Input: part model. Units: mm. Frame: model coordinates. Coordinates: 2 decimals unless noted, no trailing zeros. Order: outer loops, then holes, each group sorted by start corner. A loop starts at its lowest first (then second) coordinate and runs counter-clockwise, first axis right, second up. Notation, with made-up numbers: (79, -13) -> (137, -13) arc R18 cw to (137, 18) -> close; hole circle Ø4 at (64.5, 86). An arc over 180 degrees is marked (long way). Answer as CSV lines item,"result".
Solid Edge part; units mm, degrees
sketch "Sketch1" plane through (0, 0, 0) normal (0, -1, 0) x (1, 0, 0)
  line L0 (-92.8835, -94.8099) -> (-82.8835, -94.8099)
  line L1 (-82.8835, -94.8099) -> (-82.8835, 45.1901)
  line L2 (-82.8835, 45.1901) -> (-92.8835, 45.1901)
  line L3 (-92.8835, 45.1901) -> (-92.8835, -94.8099)
  dimension "D1" = 82.8835
  dimension "D2" = 92.8835
extrude "Protrusion1" add sketch "Sketch1" against normal blind 250
sketch "Sketch2" plane through (-82.8835, 104, 0.1901) normal (1, 0, 0) x (0, -1, 0)
  line L0 (-146, -45) -> (104, -45)
  line L1 (104, -45) -> (104, 95)
  line L2 (104, 95) -> (-146, 95)
  line L3 (-146, 95) -> (-146, -45)
  dimension "D1" = 146
  dimension "D2" = 146
extrude "Protrusion2" add sketch "Sketch2" along normal blind 10
sketch "Sketch3" plane through (-82.8835, 100, 10.1901) normal (1, 0, 0) x (0, -1, 0)
  circle A0 centre (37.5, 35) radius 2.5
  circle A1 centre (-87.5, 35) radius 2.5
extrude "Cutout1" cut sketch "Sketch3" against normal through all
extrude "ExtrudedCutout_6" [suppressed]
extrude "Cutout2" [suppressed]
sketch "Sketch4" plane through (-92.8835, 145.5, 0.1901) normal (-1, 0, 0) x (0, -1, 0)
  circle A0 centre (-31, -72) radius 5
  circle A1 centre (72, -72) radius 5
  circle A2 centre (72, -14) radius 5
  circle A3 centre (-31, -14) radius 5
extrude "Cutout3" cut sketch "Sketch4" against normal up to vertex (10 mm away)
sketch "Sketch5" plane through (-92.8835, 104, -4.8099) normal (-1, 0, 0) x (0, -1, 0)
  circle A0 centre (41.5, -20) radius 15
  circle A1 centre (-83.5, -20) radius 10
  circle A2 centre (41.5, -20) radius 10
  circle A3 centre (-83.5, -20) radius 15
extrude "ExtrudedCutout_9" cut sketch "Sketch5" against normal blind 1
hole "Hole1" at (-92.8835, 176.5, -71.8099) direction (1, 0, 0) diameter 4.917 end up to next
hole "Hole2" at (-92.8835, 73.5, -13.8099) direction (1, 0, 0) diameter 4.917 end up to next
hole "Hole3" at (-92.8835, 73.5, -71.8099) direction (1, 0, 0) diameter 4.917 end up to next
hole "Hole4" at (-92.8835, 176.5, -13.8099) direction (1, 0, 0) diameter 4.917 end up to next
hole "Hole_7" at (-92.8835, 187.5, -24.8099) direction (1, 0, 0) diameter 6.647 end up to next
hole "Hole5" at (-92.8835, 62.5, -24.8099) direction (1, 0, 0) diameter 6.647 end up to next
properties material "Aluminum, 6061-T6"
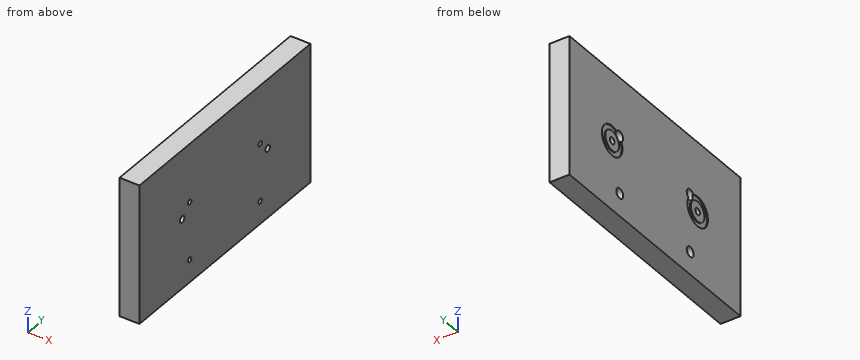
1. Contact query for a flat-ended pin moving along its axis: pin 1 (5.5 mm diameter, centred on y = 62.5, z = -24.81, fed in from -X). Output: stop coordinate, or through.
Findings:
pin 1,"passes through"
2. Ray query, line 1 along Z through (x, y) = (-88.25, 73.5); line 2 along Z through (x, y) = (-78, 176.5); line 3 along Z through (x, y) = (-92.45, 187.5). Return the intervals inside material, ascending.
Findings:
line 1,"z = -94.81 to -76.81, -66.81 to -18.81, -8.81 to 45.19"
line 2,"z = -94.81 to -74.27, -69.35 to -16.27, -11.35 to 45.19"
line 3,"z = -94.81 to -39.81, -34.81 to -28.13, -21.49 to -14.81, -9.81 to 45.19"
3. Cut plane A-A (y = 62.5). Return the cut outline in (x, z).
Findings:
outline,"(-92.88, -94.81) -> (-72.88, -94.81) -> (-72.88, -28.13) -> (-92.88, -28.13) -> (-92.88, -34.81) -> (-91.88, -34.81) -> (-91.88, -39.81) -> (-92.88, -39.81) -> close; (-92.88, -21.49) -> (-72.88, -21.49) -> (-72.88, 45.19) -> (-92.88, 45.19) -> (-92.88, -9.81) -> (-91.88, -9.81) -> (-91.88, -14.81) -> (-92.88, -14.81) -> close"
